Autodesk Inventor part; units mm, degrees
ref_plane "YZ Plane" through (0, 0, 0) normal (1, 0, 0) x (0, 1, 0)
ref_plane "XZ Plane" through (0, 0, 0) normal (0, 1, 0) x (-1, 0, 0)
ref_plane "XY Plane" through (0, 0, 0) normal (0, 0, 1) x (1, 0, 0)
sketch "Sketch1" plane through (0, 0, 0) normal (0, 1, 0) x (-1, 0, 0)
  line L0 (0, 0) -> (187, 0)
  line L1 (187, 0) -> (187, -274.11)
  line L2 (187, -274.11) -> (0, -274.11)
  line L3 (0, -274.11) -> (0, 0)
  dimension "d0" = 187
  dimension "d1" = 274.11
extrude "Extrusion1" add sketch "Sketch1" along normal blind 6.6
fillet "Fillet1" radius 7 4 edges at (0, 3.3, 0) (-187, 3.3, 0) (-187, 3.3, -274.11) (0, 3.3, -274.11)
sketch "Sketch2" plane through (0, 0, 0) normal (0, -1, 0) x (1, 0, 0)
  line L0 (-9.5, -10.055) -> (-177.5, -10.055)
  line L1 (-177.5, -10.055) -> (-177.5, -264.055)
  line L2 (-177.5, -264.055) -> (-9.5, -264.055)
  line L3 (-9.5, -264.055) -> (-9.5, -10.055)
  arc A0 (-7, -274.11) -> (0, -267.11) centre (-7, -267.11) ccw
  line L4 (0, -7) -> (0, -267.11)
  arc A1 (0, -7) -> (-7, 0) centre (-7, -7) ccw
  line L5 (-180, 0) -> (-7, 0)
  arc A2 (-180, 0) -> (-187, -7) centre (-180, -7) ccw
  line L6 (-187, -267.11) -> (-187, -7)
  arc A3 (-187, -267.11) -> (-180, -274.11) centre (-180, -267.11) ccw
  line L7 (-7, -274.11) -> (-180, -274.11)
  line L8 (-7, -7) -> (-180, -267.11) construction
  line L9 (-177.5, -10.055) -> (-9.5, -264.055) construction
  point P0 (0, 0)
  point P1 (-93.5, -137.055)
  dimension "d5" = 254
  dimension "d6" = 168
extrude "Extrusion2" add sketch "Sketch2" along normal blind 2 contours L3 L2 L1 L0
fillet "Fillet2" radius 7 4 edges at (-9.5, -1, -264.055) (-177.5, -1, -264.055) (-177.5, -1, -10.055) (-9.5, -1, -10.055)
sketch "Sketch3" plane through (0, 6.6, 0) normal (0, 1, 0) x (1, 0, 0)
  line L0 (0, 7) -> (0, 267.11)
  line L1 (0, 137.055) -> (-187, 137.055) construction
  line L2 (-187, 267.11) -> (-187, 7)
  line L3 (-7, 274.11) -> (-180, 274.11)
  line L4 (-93.5, 274.11) -> (-93.5, 0) construction
  line L5 (-180, 0) -> (-7, 0)
  circle A0 centre (-4, 137.055) radius 2
  circle A1 centre (-4, 4.5) radius 2
  circle A2 centre (-60, 4.5) radius 2
  circle A3 centre (-4, 269.61) radius 2
  line L6 (-4, 269.61) -> (-183, 269.61) construction
  line L7 (-183, 269.61) -> (-183, 4.5) construction
  line L8 (-183, 4.5) -> (-4, 4.5) construction
  line L9 (-4, 4.5) -> (-4, 269.61) construction
  circle A4 centre (-60, 269.61) radius 2
  circle A5 centre (-183, 137.055) radius 2
  circle A6 centre (-183, 4.5) radius 2
  circle A7 centre (-127, 4.5) radius 2
  circle A8 centre (-183, 269.61) radius 2
  circle A9 centre (-127, 269.61) radius 2
  point P0 (0, 0)
  dimension "d9" = 4
  dimension "d10" = 4
  dimension "d11" = 4
  dimension "d18" = 265.11
  dimension "d19" = 179
  dimension "d20" = 67
extrude "Extrusion4" cut sketch "Sketch3" against normal up to surface (6.6 mm away)
properties part number "screen_case"
The listing builds one solid part. Answer for the finished solid, in the listing's coordinates (mm). A direction names the side the tool comes from. Round coordinates to 2 decimals unless told otherwise and drop trailing zeros. Loops run counter-clockwise (first coordinate to the right, second up) from the corner with the lowest first, then second, coordinate; pieces in that order, holes last.
Q1. Given pin 1 Ø4.5 at (x, z) = (-127, -4.5) entering from +Y; pin 2 Ø0.6 at (x, y) = (-102, -1) entering from +Z (3 decimals); pin 3 Ø1.6 at (x, y) = (-80.5, -1) entering from -Z (3 decimals); pin 4 Ø0.6 at (y, z) = (-1.5, -97) entering from +X, each flat-ended and moving along its own axis, determine where each tip first touches the part or whether it passes through.
Q2. For a pull along X with two mould halves and no side action, classify faces 5 (the face through (-95, -2, -135)), 6 (the face through (-2.1, 3.3, -2)), 7 (the face through (-184.9, 3.35, -272.11)) as released by +X, released by -X, zero draft, split by the parting line, or undercut.
Q3. Find the intervals of material crossed by line 1 (Z direction, x = -60, y = 2.5); line 2 (Z direction, x = -126.5, y = 1.25); line 3 (X direction, y = 4.5, z = -137), in increasing order.
Q4. Section A-A, the plane x = -97.5 is taken. Determine the outline of the cut face in (y, z) (3 decimals), then the cut area to 3 significant figures.
Q5. Section B-B, the plane z = -104 is taken. Determine the outline of the cut face in (x, y).
Q6. Which of the six approach directions +Z, -Z, +X, -X, +Y, -Y give full straight-line access (tool end or side, diameter ignored) to faces 1 (the face through (-175.395, -1.014, -12.051)), 2 (the face through (-11.496, -1.014, -12.16)), 3 (the face through (-3, 0, -147)), 4 (the face through (-175.504, -1.014, -261.95))?
Completed:
1. pin 1: stops at y = 6.6
1. pin 2: stops at z = -10.055
1. pin 3: stops at z = -264.055
1. pin 4: stops at x = -9.5
2. face 5: zero draft
2. face 6: released by +X
2. face 7: released by -X
3. line 1: z = -274.11 to -271.61, -267.61 to -6.5, -2.5 to 0
3. line 2: z = -274.11 to -271.55, -267.67 to -6.44, -2.56 to 0
3. line 3: x = -187 to -185, -181 to -6, -2 to 0
4. outline: (-2, -264.055) - (0, -264.055) - (0, -274.11) - (6.6, -274.11) - (6.6, 0) - (0, 0) - (0, -10.055) - (-2, -10.055) - close
4. area: 2,320 mm2
5. outline: (-187, 0) - (-177.5, 0) - (-177.5, -2) - (-9.5, -2) - (-9.5, 0) - (0, 0) - (0, 6.6) - (-187, 6.6) - close
6. face 1: +Z, -X, -Y
6. face 2: +Z, +X, -Y
6. face 3: -Y
6. face 4: -Z, -X, -Y
